CAD build for the part. Positions are in the model's coordinates, mm. Coordinates: 2 decimals unless noted, no trailing zeros. Loops run counter-clockwise (first coordinate to the right, second up) from the corner with the lowest first, then second, coordinate; pieces in that order, holes last. Notation, with made-up numbers: (24, 81.5) -> (44, 81.5) arc R11 cw to (44, 87.5) -> close; hole circle Ø1 at (23, -21.5). An arc over 180 degrees is marked (long way). Write each question's results on one line, items separated by ' | '.
```python
from build123d import *

# Parameters (mm, degrees)
BOSS_EXTRUDE1_DEPTH = 10
SKETCH3_R           = 1.7
CUT_EXTRUDE1_DEPTH  = 12.874342087
FILLET2_R           = 1


with BuildPart() as part:
    # Sketch1 → Boss-Extrude1 (new body)
    with BuildSketch(Plane.XY):
        Polygon((-2.5, 0), (2.5, 0), (5, 3), (5, 4), (-5, 4), (-5, 3), align=None)
    extrude(amount=BOSS_EXTRUDE1_DEPTH)

    # Sketch3 → Cut-Extrude1 (cut, through all)
    with BuildSketch(Plane(origin=(0, 4, 0), x_dir=(1, 0, 0), z_dir=(0, 1, 0))):
        with Locations(Location((0, -5, 0), (0, 0, 270))):
            Circle(SKETCH3_R)
    extrude(amount=-CUT_EXTRUDE1_DEPTH, mode=Mode.SUBTRACT)

    # Fillet2
    # the kernel refuses this fillet: 1 mm, written as the material it takes off along each edge
    with BuildSketch(Plane(origin=(-5, 0, 10), x_dir=(0, 0, -1), z_dir=(1, 0, 0))) as fillet2_piece_1:
        with BuildLine():
            CenterArc((FILLET2_R, FILLET2_R), FILLET2_R, 180, 90)
            Line((0, FILLET2_R), (0, 0))
            Line((0, 0), (FILLET2_R, 0))
        make_face()
    extrude(amount=10, mode=Mode.SUBTRACT)
    with BuildSketch(Plane(origin=(0.899539001, -1.920553199, 10), x_dir=(-0.768221279597376, 0.6401843996644797, 0), z_dir=(0.6401843996644797, 0.768221279597376, 0))) as fillet2_piece_2:
        with BuildLine():
            CenterArc((FILLET2_R, -FILLET2_R), FILLET2_R, 90, 90)
            Line((0, -FILLET2_R), (0, 0))
            Line((0, 0), (FILLET2_R, 0))
        make_face()
    extrude(amount=8.905124838, mode=Mode.SUBTRACT)
    with BuildSketch(Plane(origin=(-6.600460999, 4.920553199, 10), x_dir=(0, 0, -1), z_dir=(0.6401843996644797, -0.768221279597376, 0))) as fillet2_piece_3:
        with BuildLine():
            CenterArc((FILLET2_R, FILLET2_R), FILLET2_R, 180, 90)
            Line((0, FILLET2_R), (0, 0))
            Line((0, 0), (FILLET2_R, 0))
        make_face()
    extrude(amount=8.905124838, mode=Mode.SUBTRACT)
    with BuildSketch(Plane(origin=(7.5, 4, 10), x_dir=(0, -1, 0), z_dir=(-1, 0, 0))) as fillet2_piece_4:
        with BuildLine():
            CenterArc((FILLET2_R, -FILLET2_R), FILLET2_R, 90, 90)
            Line((0, -FILLET2_R), (0, 0))
            Line((0, 0), (FILLET2_R, 0))
        make_face()
    extrude(amount=15, mode=Mode.SUBTRACT)
    with BuildSketch(Plane(origin=(0, 4, 5), x_dir=(0, 0, 1), z_dir=(-1, 0, 0))) as fillet2_piece_5:
        with BuildLine():
            CenterArc((1.7 + FILLET2_R, -FILLET2_R), FILLET2_R, 90, 90)
            Line((1.7 + FILLET2_R, 0), (1.7, 0))
            Line((1.7, 0), (1.7, -FILLET2_R))
        make_face()
    revolve(axis=Axis((0, 4, 5), (0, 1, 0)), mode=Mode.SUBTRACT)


solid = part.part
```
Q1. Wall check: L1, parallel to X at y = 3.8, z = 5; L2, parallel to Z at x = 1.5, y = 1.25; L3, parallel to X at y = 1.8, z = 4.75. Give the ranges that are in metal, low to high. Write a range as from..to.
Results are:
L1: -5..-2.1, 2.1..5 | L2: 0..4.2, 5.8..10 | L3: -4..-1.68, 1.68..4
Q2. Cut at B-B on z = 5. Write the cut outline in (x, y), and give its area (3 significant figures).
Results are:
outline: (-5, 3) -> (-2.5, 0) -> (-1.7, 0) -> (-1.7, 3) arc R1 ccw to (-2.7, 4) -> (-5, 4) -> close; (1.7, 0) -> (2.5, 0) -> (5, 3) -> (5, 4) -> (2.7, 4) arc R1 ccw to (1.7, 3) -> close | area: 18.5 mm^2
Q3. Pull direction Z, two halves, no side cores. Call faces 1 (the flat face through (3.732, 1.479, 4.437)), 2 (the cylindrical face through (-3.689, 1.896, 9.715)), 3 (the cylindrical face through (-0.65, 1.52, 6.57)): +Z half, -Z half, draft (parallel to the pull), parting line (faces both ways), or undercut.
Results are:
face 1: draft | face 2: +Z half | face 3: undercut
Q4. Cut at C-C on z = 1.75. Write the cut outline in (x, y), and give its area (3 significant figures).
Results are:
outline: (-5, 3) -> (-2.5, 0) -> (2.5, 0) -> (5, 3) -> (5, 4) -> (-5, 4) -> close | area: 32.5 mm^2
Q5. Drop flat-ended pins along their axis: pin 1 (1.5 mm diameter, centred on y = 2, z = 2.5, fed in from -X); pin 2 (4.5 mm diameter, centred on x = 0, z = 5, fed in from +Y). Give the stop position or say it passes through.
Results are:
pin 1: x = -4.79 | pin 2: y = 3.89
Q6. Cut at A-A on x = 0. Write the cut outline in (y, z), and give its area (3 significant figures).
Results are:
outline: (0, 0) -> (4, 0) -> (4, 2.3) arc R1 ccw to (3, 3.3) -> (0, 3.3) -> close; (0, 6.7) -> (3, 6.7) arc R1 ccw to (4, 7.7) -> (4, 9) arc R1 ccw to (3, 10) -> (1, 10) arc R1 ccw to (0, 9) -> close | area: 25.5 mm^2
